from build123d import *

# Parameters (mm, degrees)
BOX010_W        = 86
BOX010_H        = 42.2
BOX010_DEPTH    = 11.5
BOX011_W        = 82
BOX011_H        = 38.2
BOX011_DEPTH    = 9.5
SKETCH022_R     = 2.7
PAD017_DEPTH    = 6
SKETCH023_W     = 72
SKETCH023_H     = 25
POCKET005_DEPTH = 2
SKETCH024_R     = 1.7
POCKET006_DEPTH = 20


with BuildPart() as part:
    # Box010 → Box010 (join)
    with BuildSketch(Plane.XY):
        with Locations((43, 21.1)):
            Rectangle(BOX010_W, BOX010_H)
    extrude(amount=BOX010_DEPTH)

    # Box011 → Box011 (cut)
    with BuildSketch(Plane(origin=(2, 2, 2), x_dir=(1, 0, 0), z_dir=(0, 0, 1))):
        with Locations((41, 19.1)):
            Rectangle(BOX011_W, BOX011_H)
    extrude(amount=BOX011_DEPTH, mode=Mode.SUBTRACT)

    # Sketch022 → Pad017 (join)
    with BuildSketch(Plane.XY.offset(2)):
        with Locations((5.25, 36.35)):
            Circle(SKETCH022_R)
        with Locations((80.75, 36.35)):
            Circle(SKETCH022_R)
        with Locations((80.75, 5.85)):
            Circle(SKETCH022_R)
        with Locations((5.25, 5.85)):
            Circle(SKETCH022_R)
    extrude(amount=PAD017_DEPTH)

    # Sketch023 → Pocket005 (cut)
    with BuildSketch(Plane.XY):
        with Locations((43, 21.1)):
            Rectangle(SKETCH023_W, SKETCH023_H)
    extrude(amount=POCKET005_DEPTH, mode=Mode.SUBTRACT)

    # Sketch024 → Pocket006 (cut)
    with BuildSketch(Plane.XY):
        with Locations((5.25, 36.35)):
            Circle(SKETCH024_R)
        with Locations((80.75, 36.35)):
            Circle(SKETCH024_R)
        with Locations((80.75, 5.85)):
            Circle(SKETCH024_R)
        with Locations((5.25, 5.85)):
            Circle(SKETCH024_R)
    extrude(amount=POCKET006_DEPTH, mode=Mode.SUBTRACT)


solid = part.part
Check sheet for the modelled part. Datum: model origin and axes. Units: mm. A direction names the side the tool comes from. Round coordinates to 2 decimals unless told otherwise and drop trailing zeros. Loops run counter-clockwise (first coordinate to the right, second up) from the corner with the lowest first, then second, coordinate; pieces in that order, holes last. Notation, with made-up numbers: (-21, -0.5) -> (-1, -0.5) arc R13 ccw to (-1, 7.5) -> close; hole circle Ø3 at (75, 47). An arc over 180 degrees is marked (long way). Put each result on its own line as item: value. Start each with the question number.
1. Section check D-D (x = 5.25). Enter the section's corners in (y, z), plus the area to 3 significant figures.
2. Section check B-B (x = 72.5). Enter the section's corners in (y, z).
3. Gauge pin test, flat ends, axial feed: pin 1 (4.5 mm diameter, centred on x = 4.5, y = 36.5, fed in from +Z); pin 2 (19 mm diameter, centred on x = 57, y = 23.5, fed in from +Z). Record the tip position at first contact, or that the pin passes through.
4. Access from +Z, -Z, +X, -X, +Y, -Y to the whole of each face (thin tool, end or side, straight path). Record for faces 1 (the face through (86, 21, 6)), 2 (the face through (79, 21, 1)), 3 (the face through (2, 21, 7)).
5. Section check A-A (z = 6). Give the number of separate pieces and of enclosed holes in the cut face, plus the area to 3 significant figures.
6. Scan lines: probe 1 along Y at (x, z) = (80.75, 3.25); probe 2 along Y at (x, z) = (7.5, 9.5); probe 3 along Y at (x, z) = (26, 0.75). Record each from-to range of solid material in increasing order.
7. Section check C-C (y = 27). Enter the section's corners in (x, z).
8. Draft check along X on faces 4 (the face through (0, 21, 6)), 5 (the face through (83, 36, 8)), 6 (the face through (49, 8, 2)), 7 (the face through (42, 7, 0)). Enter one of: +X half, -X half, draft (parallel to the pull), parting line (faces both ways), or undercut.
Findings:
1. outline: (0, 0) -> (4.15, 0) -> (4.15, 8) -> (3.15, 8) -> (3.15, 2) -> (2, 2) -> (2, 11.5) -> (0, 11.5) -> close; (7.55, 0) -> (34.65, 0) -> (34.65, 8) -> (33.65, 8) -> (33.65, 2) -> (8.55, 2) -> (8.55, 8) -> (7.55, 8) -> close; (38.05, 0) -> (42.2, 0) -> (42.2, 11.5) -> (40.2, 11.5) -> (40.2, 2) -> (39.05, 2) -> (39.05, 8) -> (38.05, 8) -> close
1. area: 133 mm^2
2. outline: (0, 0) -> (8.6, 0) -> (8.6, 2) -> (2, 2) -> (2, 11.5) -> (0, 11.5) -> close; (33.6, 0) -> (42.2, 0) -> (42.2, 11.5) -> (40.2, 11.5) -> (40.2, 2) -> (33.6, 2) -> close
3. pin 1: stops at z = 8
3. pin 2: passes through
4. face 1: +Z, -Z, +X, +Y, -Y
4. face 2: +Z, -Z
4. face 3: +Z
5. separate pieces: 5
5. enclosed holes: 5
5. area: 552 mm^2
6. probe 1: y = 0 to 2, 3.15 to 4.15, 7.55 to 8.55, 33.65 to 34.65, 38.05 to 39.05, 40.2 to 42.2
6. probe 2: y = 0 to 2, 40.2 to 42.2
6. probe 3: y = 0 to 8.6, 33.6 to 42.2
7. outline: (0, 0) -> (7, 0) -> (7, 2) -> (2, 2) -> (2, 11.5) -> (0, 11.5) -> close; (79, 0) -> (86, 0) -> (86, 11.5) -> (84, 11.5) -> (84, 2) -> (79, 2) -> close
8. face 4: -X half
8. face 5: undercut
8. face 6: undercut
8. face 7: draft
